```python
from build123d import *

# Parameters (mm, degrees)
F0_W     = 300
F0_H     = 2180
F1_DEPTH = 46
F0_W_2   = 294
F0_H_2   = 209
F0_R     = 3.5
F0_W_3   = 220
F0_H_3   = 135
F0_W_4   = 37
F0_H_4   = 126
F0_H_5   = 1492
F0_H_6   = 1418
F2_DEPTH = 3


with BuildPart() as f1:
    # F0 (on Front) → F1 (new body)
    with BuildSketch(Plane.XZ):
        Rectangle(F0_W, F0_H)
        Polygon((-147, 878), (-147, 1087), (147, 1087), (147, 878), (147, 875), (147, 749), (147, 746), (147, -746), (147, -749), (147, -875), (147, -878), (147, -1087), (-147, -1087), (-147, -878), (-147, -875), (-147, -749), (-147, -746), (-147, 746), (-147, 749), (-147, 875), align=None, mode=Mode.SUBTRACT)
        Polygon((147, -746), (-147, -746), (-147, -749), (-110, -749), (110, -749), (147, -749), align=None)
        Polygon((-110, -875), (-147, -875), (-147, -878), (147, -878), (147, -875), (110, -875), align=None)
        Polygon((-110, 749), (-147, 749), (-147, 746), (147, 746), (147, 749), (110, 749), align=None)
        Polygon((147, 878), (-147, 878), (-147, 875), (-110, 875), (110, 875), (147, 875), align=None)
    extrude(amount=F1_DEPTH)

    # F0 (on Front) → F2 (join)
    with BuildSketch(Plane.XZ):
        with Locations((0, 982.5)):
            Rectangle(F0_W_2, F0_H_2)
        with Locations((-130, 946)):
            Circle(F0_R, mode=Mode.SUBTRACT)
        with Locations((-130, 1026)):
            Circle(F0_R, mode=Mode.SUBTRACT)
        with Locations((0, 982.5)):
            Rectangle(F0_W_3, F0_H_3, mode=Mode.SUBTRACT)
        with Locations((0, 1070)):
            Circle(F0_R, mode=Mode.SUBTRACT)
        with Locations((130, 945)):
            Circle(F0_R, mode=Mode.SUBTRACT)
        with Locations((130, 1025)):
            Circle(F0_R, mode=Mode.SUBTRACT)
        with Locations((-128.5, 812)):
            Rectangle(F0_W_4, F0_H_4)
        with Locations((-130, 759)):
            Circle(F0_R, mode=Mode.SUBTRACT)
        with Locations((-130, 839)):
            Circle(F0_R, mode=Mode.SUBTRACT)
        with Locations((128.5, 812)):
            Rectangle(F0_W_4, F0_H_4)
        with Locations((130, 758)):
            Circle(F0_R, mode=Mode.SUBTRACT)
        with Locations((130, 838)):
            Circle(F0_R, mode=Mode.SUBTRACT)
        Rectangle(F0_W_2, F0_H_5)
        with Locations((-130, -648)):
            Circle(F0_R, mode=Mode.SUBTRACT)
        with Locations((-130, -536)):
            Circle(F0_R, mode=Mode.SUBTRACT)
        with Locations((-130, -446)):
            Circle(F0_R, mode=Mode.SUBTRACT)
        with Locations((-130, -336)):
            Circle(F0_R, mode=Mode.SUBTRACT)
        with Locations((-130, -246)):
            Circle(F0_R, mode=Mode.SUBTRACT)
        with Locations((-130, -136)):
            Circle(F0_R, mode=Mode.SUBTRACT)
        with Locations((-130, -46)):
            Circle(F0_R, mode=Mode.SUBTRACT)
        with Locations((130, -645)):
            Circle(F0_R, mode=Mode.SUBTRACT)
        with Locations((130, -533)):
            Circle(F0_R, mode=Mode.SUBTRACT)
        with Locations((130, -443)):
            Circle(F0_R, mode=Mode.SUBTRACT)
        with Locations((130, -333)):
            Circle(F0_R, mode=Mode.SUBTRACT)
        with Locations((130, -243)):
            Circle(F0_R, mode=Mode.SUBTRACT)
        with Locations((130, -133)):
            Circle(F0_R, mode=Mode.SUBTRACT)
        with Locations((130, -43)):
            Circle(F0_R, mode=Mode.SUBTRACT)
        with Locations((-130, 64)):
            Circle(F0_R, mode=Mode.SUBTRACT)
        with Locations((-130, 154)):
            Circle(F0_R, mode=Mode.SUBTRACT)
        with Locations((-130, 264)):
            Circle(F0_R, mode=Mode.SUBTRACT)
        with Locations((-130, 354)):
            Circle(F0_R, mode=Mode.SUBTRACT)
        with Locations((-130, 464)):
            Circle(F0_R, mode=Mode.SUBTRACT)
        with Locations((-130, 554)):
            Circle(F0_R, mode=Mode.SUBTRACT)
        with Locations((-130, 664)):
            Circle(F0_R, mode=Mode.SUBTRACT)
        Rectangle(F0_W_3, F0_H_6, mode=Mode.SUBTRACT)
        with Locations((130, 67)):
            Circle(F0_R, mode=Mode.SUBTRACT)
        with Locations((130, 157)):
            Circle(F0_R, mode=Mode.SUBTRACT)
        with Locations((130, 267)):
            Circle(F0_R, mode=Mode.SUBTRACT)
        with Locations((130, 357)):
            Circle(F0_R, mode=Mode.SUBTRACT)
        with Locations((130, 467)):
            Circle(F0_R, mode=Mode.SUBTRACT)
        with Locations((130, 557)):
            Circle(F0_R, mode=Mode.SUBTRACT)
        with Locations((130, 667)):
            Circle(F0_R, mode=Mode.SUBTRACT)
        with Locations((-128.5, -812)):
            Rectangle(F0_W_4, F0_H_4)
        with Locations((-130, -839.5)):
            Circle(F0_R, mode=Mode.SUBTRACT)
        with Locations((-130, -759.5)):
            Circle(F0_R, mode=Mode.SUBTRACT)
        with Locations((128.5, -812)):
            Rectangle(F0_W_4, F0_H_4)
        with Locations((130, -836.5)):
            Circle(F0_R, mode=Mode.SUBTRACT)
        with Locations((130, -756.5)):
            Circle(F0_R, mode=Mode.SUBTRACT)
        with Locations((0, -982.5)):
            Rectangle(F0_W_2, F0_H_2)
        with Locations((-130, -1026.5)):
            Circle(F0_R, mode=Mode.SUBTRACT)
        with Locations((-130, -946.5)):
            Circle(F0_R, mode=Mode.SUBTRACT)
        with Locations((0, -1070)):
            Circle(F0_R, mode=Mode.SUBTRACT)
        with Locations((0, -982.5)):
            Rectangle(F0_W_3, F0_H_3, mode=Mode.SUBTRACT)
        with Locations((130, -1023.5)):
            Circle(F0_R, mode=Mode.SUBTRACT)
        with Locations((130, -943.5)):
            Circle(F0_R, mode=Mode.SUBTRACT)
    extrude(amount=F2_DEPTH)


solid = f1.part
```
Check sheet for the modelled part. Datum: model origin and axes. Units: mm. A direction names the side the tool comes from. Round coordinates to 2 decimals unless told otherwise and drop trailing zeros. Order: outer loops, then holes, each group sorted by start corner. A loop starts at its lowest first (then second) coordinate and runs counter-clockwise, first axis right, second up.
1) Section check A-A (z = 636). Record the boundary of the cut face in (x, y).
2) Go/stop test with flat-tipped pins: pin 1 Ø4 at (x, z) = (109, -605.5) entering from -Y; pin 2 Ø11 at (x, z) = (-130, -246) entering from +Y. Record where each tip stops, or that it passes through.
3) Tool access check on faces 1 (the flat face through (-135, 0, 15)), 2 (the flat face through (-2, -24, -878)). Record the directions out of +Z, -Z, +X, -X, +Y, -Y that give a thin tool (end or side, any length) a straight path to the whole face; none if there is none.
4) Section check C-C (x = 24.5). Give the number of separate pieces and of enclosed holes in the cut face, and give its area (3 significant figures).
5) Section check B-B (y = -25). Record the boundary of the cut face in (x, z).
6) Mould release check, pull along X, two halves, no side actions. Record for faces 3 (the flat face through (-150, -23, -15)), 4 (the flat face through (2, -24, -1087)), 5 (the flat face through (-2, -23, 1090)): +X half, -X half, draft (parallel to the pull), parting line (faces both ways), or undercut.
7) Scan lines: line 1 (Z direction, x = -49, y = -10.5); line 2 (X direction, y = -23, z = -408); line 3 (X direction, y = -2, z = -333). Record each from-to range of solid material in increasing order.
Result:
1. outline: (-150, -46) - (-147, -46) - (-147, -3) - (-110, -3) - (-110, 0) - (-150, 0) - close; (110, -3) - (147, -3) - (147, -46) - (150, -46) - (150, 0) - (110, 0) - close
2. pin 1: stops at y = -3
2. pin 2: stops at y = 0
3. face 1: +Z, -Z, +X, -X, +Y
3. face 2: -Y
4. separate pieces: 6
4. enclosed holes: 0
4. area: 1,490 mm2
5. outline: (-150, -1090) - (150, -1090) - (150, 1090) - (-150, 1090) - close; hole (-147, -1087) - (147, -1087) - (147, -878) - (-147, -878) - close; hole (-147, -875) - (147, -875) - (147, -749) - (-147, -749) - close; hole (-147, -746) - (147, -746) - (147, 746) - (-147, 746) - close; hole (-147, 749) - (147, 749) - (147, 875) - (-147, 875) - close; hole (-147, 878) - (147, 878) - (147, 1087) - (-147, 1087) - close
6. face 3: -X half
6. face 4: undercut
6. face 5: draft
7. line 1: z = -1090 to -1087, -878 to -875, -749 to -746, 746 to 749, 875 to 878, 1087 to 1090
7. line 2: x = -150 to -147, 147 to 150
7. line 3: x = -150 to -131.8, -128.2 to -110, 110 to 126.5, 133.5 to 150
